The listing builds one solid part. Answer for the finished solid, in the listing's coordinates (mm). A direction names the side the tool comes from. Coordinates: 2 decimals unless noted, no trailing zeros. Write each loop counter-clockwise with the first axis right and the second up, starting at its lowest first coordinate (ties: lowest second). Pieces come first, ordered by that corner, then holes.
Autodesk Inventor part; units mm, degrees
ref_plane "YZ Plane" through (0, 0, 0) normal (1, 0, 0) x (0, 1, 0)
ref_plane "XZ Plane" through (0, 0, 0) normal (0, 1, 0) x (-1, 0, 0)
ref_plane "XY Plane" through (0, 0, 0) normal (0, 0, 1) x (1, 0, 0)
sketch "Sketch1" plane through (0, 0, 0) normal (0, 0, 1) x (1, 0, 0)
  circle A0 centre (0, 0) radius 10
  dimension "d0" = 20
extrude "Extrusion1" add sketch "Sketch1" along normal blind 1
sketch "Sketch2" plane through (0, 0, 1) normal (0, 0, 1) x (1, 0, 0)
  circle A0 centre (0, 0) radius 8.5
  dimension "d3" = 17
extrude "Extrusion2" add sketch "Sketch2" along normal blind 2
sketch "Sketch3" plane through (0, 0, 3) normal (0, 0, 1) x (1, 0, 0)
  circle A0 centre (0, 0) radius 9.8227
extrude "Extrusion3" add sketch "Sketch3" along normal blind 1
sketch "Sketch4" plane through (0, 0, 4) normal (0, 0, 1) x (1, 0, 0)
  circle A0 centre (0, 0) radius 4.5
  line L0 (-3.25, 1.75) -> (3.25, 1.75)
  line L1 (3.25, 1.75) -> (3.25, -1.75)
  line L2 (3.25, -1.75) -> (-3.25, -1.75)
  line L3 (-3.25, -1.75) -> (-3.25, 1.75)
  dimension "d8" = 9
  dimension "d9" = 3.5
  dimension "d10" = 6.5
  dimension "d11" = 1.75
  dimension "d12" = 3.25
extrude "Extrusion4" add sketch "Sketch4" along normal blind 7
sketch "Sketch5" plane through (0, 0, 0) normal (0, 0, -1) x (-1, 0, 0)
  point P0 (0, 0)
sketch "Sketch6" plane through (0, 0, 11) normal (0, 0, 1) x (1, 0, 0)
  circle A0 centre (0, 0) radius 4.5
extrude "Extrusion5" cut sketch "Sketch6" against normal blind 7
sketch "Sketch7" plane through (0, 0, 4) normal (0, 0, 1) x (1, 0, 0)
  line L0 (-13.328, 0) -> (12.5041, 0)
  line L1 (12.5041, 0) -> (12.5041, -10.2387)
  line L2 (12.5041, -10.2387) -> (-13.328, -10.2387)
  line L3 (-13.328, -10.2387) -> (-13.328, 0)
  point P0 (0, 0)
extrude "Extrusion6" cut sketch "Sketch7" against normal blind 10
sketch "Sketch8" plane through (-9.8227, 0, 4) normal (0, -1, 0) x (1, 0, 0)
  line L0 (19.8227, -3) -> (-0.1773, -3)
  line L1 (1.3199, -0.999) -> (18.3844, -0.999)
  line L2 (18.3844, -0.999) -> (18.3844, -3)
  line L3 (18.3844, -3) -> (1.3199, -3)
  line L4 (1.3199, -3) -> (1.3199, -0.999)
  point P0 (9.8227, -4)
extrude "Extrusion7" cut sketch "Sketch8" against normal blind 3
properties part number "Top Holder"
1. Section C-C on y = 4 is taken. Give the vertices of the cut face in (x, z).
Results found:
outline: (-9.17, 0) - (9.17, 0) - (9.17, 1) - (7.5, 1) - (7.5, 3) - (8.97, 3) - (8.97, 4) - (-8.97, 4) - (-8.97, 3) - (-7.5, 3) - (-7.5, 1) - (-9.17, 1) - close
2. A tool of negligible diameter and unlimited length cuts with its end or side. For faces 4 (the flat face through (0.1, 2.7, 1)), 5 (the cylindrical face through (-0.1, 8.5, 2)), 6 (the cylindrical face through (-0.2, 10, 0.5)), 7 (the cylindrical face through (-0.22, 9.82, 3.49)), 8 (the flat face through (0, 1, 3.001)), from which of +Z, -Z, +X, -X, +Y, -Y can it reach the whole face along a straight path? Write none if from no direction.
Results found:
face 4: none
face 5: +Y
face 6: +Z, -Z, +Y
face 7: +Z, +Y
face 8: +X, -X, -Y
3. Section B-B on x = 0 is taken. Give the vertices of the cut face in (y, z), then the cut area to 3 significant figures.
Results found:
outline: (0, 0) - (10, 0) - (10, 1) - (8.5, 1) - (8.5, 3) - (9.82, 3) - (9.82, 4) - (0, 4) - (0, 3) - (3, 3) - (3, 1) - (0, 1) - close
area: 30.8 mm2
4. Section D-D on z = 2.8 is taken. Give the vertices of the cut face in (x, y).
Results found:
outline: (-7.95, 3) - (7.95, 3) arc R8.5 ccw to start
5. For a pull along Z with two mould halves and no side action, classify faces 1 (the flat face through (0, 4, 4)), 2 (the flat face through (0, 4, 0)), 3 (the flat face through (0, 9, 3)) as pulls with the +Z half, pulls with the -Z half, needs draft (parallel to the pull), parting line crosses it, or undercut.
Results found:
face 1: pulls with the +Z half
face 2: pulls with the -Z half
face 3: undercut
6. A flat-ended cylindrical pin translates along its axis: P1, Ø0.6, axis at x = 3, z = 2.5, coming from the -Y side. Find the tip coordinate at first contact, or state that the pin passes through.
Results found:
P1: stops at y = 3
7. Find the intervals of material crossed by L1, parallel to Z at x = -3.5, y = 2; L2, parallel to Y at x = 0, z = 0.8; L3, parallel to Y at x = 4.75, z = 1.2, in increasing order.
Results found:
L1: z = 0 to 1, 3 to 4
L2: y = 0 to 10
L3: y = 3 to 7.05
